Can you work these out from the model? Positions are in its coordinate system, mm. Coordinates: 2 decimals unless noted, no trailing zeros. Order: outer loops, then holes, each group sorted by start corner. A loop starts at its lowest first (then second) coordinate and runs counter-clockwise, first axis right, second up. Notation, with made-up numbers: (76, -17.75) - (106, -17.75) arc R8 ccw to (106, -6.75) - close; hole circle Ø2 at (46.5, -34.75). An arc over 180 degrees is marked (long way). Return JSON: item names as keys, results as strings. Group by question number.
1) Imagine slicing it at D-D (x = -9.5). Write out the boundary of the cut face in (y, z).
2) For pin 1 Ø2 at (y, z) = (18.5, -6) entering from +X; pin 2 Ø4 at (x, y) = (0, 0) entering from +Z; pin 3 Ø1 at (x, y) = (7, -17) entering from +Z, each with a flat end and sliding along its axis, tell me the tip position at first contact or that it passes through.
3) If I drill on line 1 along Z through (x, y) = (-9.5, -18.5); line 2 along Z through (x, y) = (16, -22.5); line 3 along X through (y, z) = (-12, 8), over which ranges is the centre line in solid material (lowest first)?
4) Imagine slicing it at C-C (y = -8). Write out the boundary of the cut face in (x, z).
5) Imagine slicing it at A-A (y = 0). Write out the boundary of the cut face in (x, z).
```python
from build123d import *

# Parameters (mm, degrees)
F2_T     = -2
F3_R     = 2.5
F4_DEPTH = 32.501


with BuildPart() as f1:
    # F0 (on Top) → F1 (revolve)
    with BuildSketch(Plane.XY):
        with BuildLine():
            ThreePointArc((32.5, 0), (0, 32.5), (-32.5, 0))
            Line((-32.5, 0), (32.5, 0))
        make_face()
    revolve(axis=Axis((0, 0, 0), (1, 0, 0)))

    # F2 (hollow: no face is removed)
    offset(amount=F2_T, mode=Mode.SUBTRACT)

    # F3 (on Top) → F4 (cut, through all)
    with BuildSketch(Plane.XY):
        Circle(F3_R)
    extrude(amount=-F4_DEPTH, mode=Mode.SUBTRACT)


solid = f1.part
```
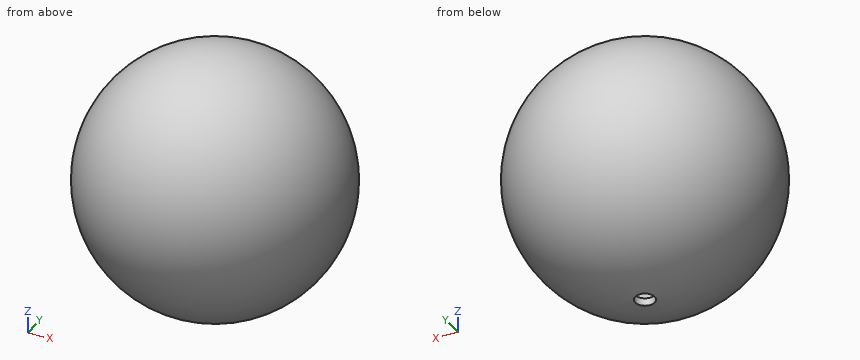
Calculated:
{
 "1": {"outline": "circle Ø62.16 at (0, 0); hole circle Ø57.97 at (0, 0)"},
 "2": {"pin 1": "x = 26.76", "pin 2": "z = 32.5", "pin 3": "z = 27.14"},
 "3": {"line 1": "-24.97 to -22.31, 22.31 to 24.97", "line 2": "-17.15 to -12.96, 12.96 to 17.15", "line 3": "-29.12 to -26.87, 26.87 to 29.12"},
 "4": {"outline": "circle Ø63 at (0, 0); hole circle Ø58.86 at (0, 0)"},
 "5": {"outline": "(-2.5, -32.4) - (-2.5, -30.4) arc R30.5 cw (long way) to (2.5, -30.4) - (2.5, -32.4) arc R32.5 ccw (long way) to start"}
}
